```python
from build123d import *

# Parameters (mm, degrees)
F0_W     = 76.2
F0_H     = 50.8
F1_DEPTH = 2.54
F3_DEPTH = 3.81
F4_SIZE  = 1.778


with BuildPart() as f1:
    # F0 (on Top) → F1 (new body)
    with BuildSketch(Plane.XY):
        with Locations((2.905123, -2.270125)):
            Rectangle(F0_W, F0_H)
    extrude(amount=F1_DEPTH)

    # F2 (on face) → F3 (join)
    with BuildSketch(Plane.XY.offset(2.54)):
        Polygon((37.957123, 20.081875), (-32.146877, 20.081875), (-32.146877, -24.622125), (37.957123, -24.622125), (37.957123, 4.333875), align=None)
    extrude(amount=F3_DEPTH)

    # F4
    f4_edges = [f1.edges().sort_by_distance(p)[0] for p in [
        (2.905123, -24.622125, 6.35),
        (-32.146877, -2.270125, 6.35),
        (37.957123, -2.270125, 6.35),
        (2.905123, 20.081875, 6.35),
    ]]
    chamfer(f4_edges, length=F4_SIZE)


solid = f1.part
```
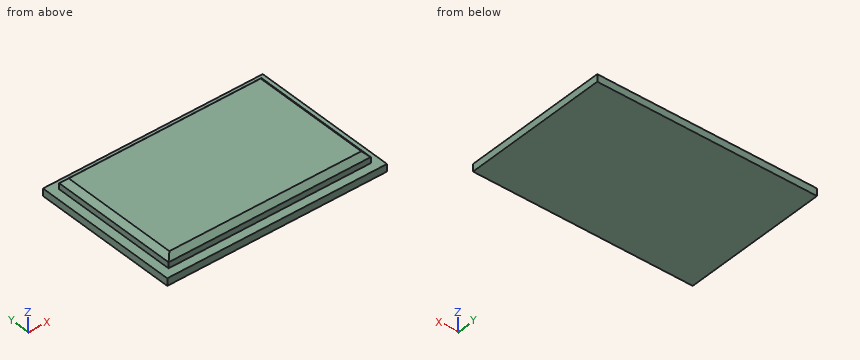
Part model, mm, in its own coordinate system. Round coordinates to 2 decimals unless told otherwise and drop trailing zeros. Order: outer loops, then holes, each group sorted by start corner. A loop starts at its lowest first (then second) coordinate and runs counter-clockwise, first axis right, second up. Notation, with made-up numbers: M -6,89.5 L 44,89.5 A22 ccw 44,122.5 Z; hole C 38,56 d11. An arc over 180 degrees is marked long. Answer in a Markdown table with one row per item. Add a question column.
Q1. Cut at A-A on x = -18.5. Give the cut face in (y, z), and give its area (3 significant figures).
Q2. Pin check, flat tips, straight feed: pin 1 (1.6 mm diameter, centred on y = -5.5, z = 3.5, fed in from -X); pin 2 (0.6 mm diameter, centred on x = -0.5, z = 3.5, fed in from -Y); pin 3 (2 mm diameter, centred on y = -8, z = 4, fed in from +X). Stop position of each tip, or through.
Q3. Wall check: L1, parallel to Y at x = 29.5, z = 2.75; L2, parallel to X at y = -19, z = 4.5; L3, parallel to Z at x = -20, y = 18.5. Give the ranges that are in metal, low to high. Write a range as from..to.
Q4. Cut at C-C on z = 3.75. Give the cut face in (x, y).
Q5. Cut at B-B on y = 8.5. Give the cut face in (x, z), and give its area (3 significant figures).
Established:
| question | item | result |
|---|---|---|
| 1 | outline | M -27.67,0 L 23.13,0 L 23.13,2.54 L 20.08,2.54 L 20.08,4.57 L 18.3,6.35 L -22.84,6.35 L -24.62,4.57 L -24.62,2.54 L -27.67,2.54 Z |
| 1 | area | 296 mm2 |
| 2 | pin 1 | stops at x = -32.15 |
| 2 | pin 2 | stops at y = -24.62 |
| 2 | pin 3 | stops at x = 37.96 |
| 3 | L1 | y = -24.62..20.08 |
| 3 | L2 | x = -32.15..37.96 |
| 3 | L3 | z = 0..6.15 |
| 4 | outline | M -32.15,-24.62 L 37.96,-24.62 L 37.96,20.08 L -32.15,20.08 Z |
| 5 | outline | M -35.19,0 L 41.01,0 L 41.01,2.54 L 37.96,2.54 L 37.96,4.57 L 36.18,6.35 L -30.37,6.35 L -32.15,4.57 L -32.15,2.54 L -35.19,2.54 Z |
| 5 | area | 457 mm2 |
